Input: part model. Units: mm. Frame: model coordinates. A direction names the side the tool comes from. Round coordinates to 2 decimals unless told otherwise and drop trailing zeros. Order: outer loops, then holes, each group sorted by start corner. A loop starts at its lowest first (then second) coordinate and runs counter-clockwise, first axis right, second up. Notation, with made-up numbers: (49, 66.5) -> (56, 66.5) arc R13 ccw to (56, 81.5) -> close; hole circle Ø10 at (81.5, 69). An arc over 180 degrees is marked (long way). Answer as CSV lines item,"result". Start each with the question number.
1) Mould query, pull axis X, two halves, no side actions, for faces 6 (the face through (-3, -3, 2)), 7 (the face through (0, -7, 1)), 8 (the face through (-6.764, -1.925, 0.789)). Classes: +X half, -X half, draft (parallel to the pull), parting line (faces both ways), or undercut.
2) Section query C-C, the plane z = 1.2. Output: boundary loops of the cut face in (x, y), and give its area (3 significant figures).
3) Section query D-D, the plane x = -4.75. Output: boundary loops of the cut face in (y, z), and give its area (3 significant figures).
4) Line query: L1, parallel to Z at x = -8.25, y = -7.5; L2, parallel to Y at x = -7.25, z = 0.65; L3, parallel to Y at x = -5, z = 2.1. Output: solid intervals per line, ascending.
5) Access query for faces 1 (the face through (-0.7, -4, 2)), 2 (the face through (-3, -4, 2.6)), 3 (the face through (-3, -5.4, 2)), 4 (the face through (-5.1, -4, 2)), 5 (the face through (-5, -13.35, 1)). Directions: +Z, -Z, +X, -X, +Y, -Y. A direction counts if a zero-diameter tool reaches every point of the face in a straight line with its end or side. Return the directions, or none.
6) First-contact query: P1, Ø1.1, axis at x = -2.5, z = 2.5, coming from the -Y side. Flat tip, straight axial feed; report the tip coordinate or a pass-through.
7) Section query B-B, the plane x = -8.15. Output: boundary loops of the cut face in (y, z), and give its area (3 significant figures).
8) Section query A-A, the plane y = -2.5. Output: boundary loops of the cut face in (x, z), and give its area (3 significant figures).
Autodesk Inventor part; units mm, degrees
ref_plane "YZ Plane" through (0, 0, 0) normal (1, 0, 0) x (0, 1, 0)
ref_plane "XZ Plane" through (0, 0, 0) normal (0, 1, 0) x (-1, 0, 0)
ref_plane "XY Plane" through (0, 0, 0) normal (0, 0, 1) x (1, 0, 0)
sketch "Náčrt1" plane through (0, 0, 0) normal (0, 0, 1) x (1, 0, 0)
  line L0 (-10.65, 0) -> (0, 0)
  line L1 (0, 0) -> (0, -13.35)
  line L2 (0, -13.35) -> (-10.65, -13.35)
  line L3 (-10.65, -13.35) -> (-10.65, 0)
  circle A0 centre (-8.15, -2.5) radius 1.5
  dimension "d0" = 10.65
  dimension "d1" = 13.35
  dimension "d2" = 3
  dimension "d3" = 1
  dimension "d4" = 1
extrude "Vysunutí1" add sketch "Náčrt1" along normal blind 1.6
sketch "Náčrt2" plane through (0, 0, 1.6) normal (0, 0, 1) x (1, 0, 0)
  line L0 (-5.1, -3) -> (-0.7, -3)
  line L1 (-0.7, -3) -> (-0.7, -5.4)
  line L2 (-0.7, -5.4) -> (-5.1, -5.4)
  line L3 (-5.1, -5.4) -> (-5.1, -3)
  point P0 (0, 0)
  dimension "d7" = 2.4
  dimension "d8" = 4.4
  dimension "d9" = 3
  dimension "d10" = 0.7
extrude "Vysunutí2" add sketch "Náčrt2" along normal blind 1
sketch "Náčrt3" plane through (0, 0, 2.6) normal (0, 0, 1) x (1, 0, 0)
  circle A0 centre (-4.365, -4.2) radius 0.2
  circle A1 centre (-1.365, -4.2) radius 0.1
  line L0 (-5.1, -3) -> (-5.1, -5.4)
  line L1 (-0.7, -5.4) -> (-0.7, -3)
  point P0 (0, 0)
  point P1 (-5.1, -4.2)
  point P2 (-0.7, -4.2)
  dimension "d13" = 0.4
  dimension "d14" = 0.2
  dimension "d16" = 0.665
  dimension "d17" = 3
extrude "Vysunutí3" cut sketch "Náčrt3" against normal blind 0.1
properties part number "senzor"
Findings:
1,face 6,"draft"
1,face 7,"+X half"
1,face 8,"undercut"
2,outline,"(-10.65, -13.35) -> (0, -13.35) -> (0, 0) -> (-10.65, 0) -> close; hole circle Ø3 at (-8.15, -2.5)"
2,area,"135 mm^2"
3,outline,"(-13.35, 0) -> (0, 0) -> (0, 1.6) -> (-3, 1.6) -> (-3, 2.6) -> (-5.4, 2.6) -> (-5.4, 1.6) -> (-13.35, 1.6) -> close"
3,area,"23.8 mm^2"
4,L1,"z = 0 to 1.6"
4,L2,"y = -13.35 to -3.7, -1.3 to 0"
4,L3,"y = -5.4 to -3"
5,face 1,"+Z, +X, +Y, -Y"
5,face 2,"+Z, +X, -X, +Y, -Y"
5,face 3,"+Z, +X, -X, -Y"
5,face 4,"+Z, -X, +Y, -Y"
5,face 5,"+Z, -Z, +X, -X, -Y"
6,P1,"stops at y = -5.4"
7,outline,"(-13.35, 0) -> (-4, 0) -> (-4, 1.6) -> (-13.35, 1.6) -> close; (-1, 0) -> (0, 0) -> (0, 1.6) -> (-1, 1.6) -> close"
7,area,"16.6 mm^2"
8,outline,"(-10.65, 0) -> (-9.65, 0) -> (-9.65, 1.6) -> (-10.65, 1.6) -> close; (-6.65, 0) -> (0, 0) -> (0, 1.6) -> (-6.65, 1.6) -> close"
8,area,"12.2 mm^2"
